For this review, take the finished solid that the model builds, in its own axes (mm). A direction names the side the tool comes from. Coordinates: 2 decimals unless noted, no trailing zeros. Order: outer loops, then holes, each group sorted by start corner. A loop starts at its lowest first (then second) coordinate and runs counter-clockwise, first axis right, second up. Notation, with made-up numbers: (-32, 14.5) -> (-1, 14.5) arc R30 ccw to (-1, 36.5) -> close; hole circle Ø4 at (-24, -24). An arc over 180 degrees is marked (long way). Return JSON: item names as keys, results as strings. Group by question number.
Item 1: Machinability: for faces 4 (the flat face through (-21.576, -30.4, 34.3)), 5 (the flat face through (0, -30.8, 0)), 6 (the flat face through (0, 1.336, 20)), 7 (the flat face through (0, -26, 33.65)), 8 (the flat face through (-21.576, -30.4, -34.3)), which of the approach directions +Z, -Z, +X, -X, +Y, -Y give a long, thin tool a straight path to every point of the face, cutting with its end or side? Answer none if there is none.
Item 2: Take a section at B-B (z = -38.75). Write out the cut boundary in (x, y) (3 decimals), then the cut area to 3 significant figures.
Item 3: Insertion check: pin 1 (8 mm diameter, centred on x = 4, z = 39.5, fed in from +Y); pin 2 (2 mm diameter, centred on x = -11, z = -9, fed in from +Y); pin 3 (0.7 mm diameter, centred on x = 2.5, z = -32, fed in from +Y). Each pin has a flat end and moves straight along its axis. Give the tip position at first contact, or say it passes through.
Item 4: For line 1 along X through (y, z) = (-31.1, 38.75) (3 decimals); line 2 along Y through (x, z) = (0, 16); line 3 along Y through (x, z) = (-16, -16), list the stretches that pass through material, from the lowest coordinate up.
Item 5: Draft analysis for pull direction Z (two halves, no side actions). For faces 1 (the cylindrical face through (13.947, -31.291, -40.505)), 2 (the flat face through (0, -30.15, 39)), 3 (the flat face through (0, -31, 43.7)), state which applies: +Z half, -Z half, draft (parallel to the pull), parting line (faces both ways), or undercut.
Item 6: Take a section at C-C (y = -27). Write out the cut boundary in (x, z).
Item 7: Take a section at A-A (z = 38.75). Write out the cut boundary in (x, y) (3 decimals), then the cut area to 3 significant figures.
Item 8: Take a section at D-D (x = 19). Write out the cut boundary in (y, z).
```python
from build123d import *

# Parameters (mm, degrees)
SKETCH1_W                = 46.2
SKETCH1_H                = 60
BOSS_EXTRUDE1_DEPTH      = 30.8
FILLET1_R                = 1.524
BOSS_EXTRUDE2_DEPTH      = 6
BOSS_EXTRUDE2_DEPTH_BACK = 12.07
SKETCH2_R                = 8.849999953
SKETCH3_R                = 5.849999953
CUT_EXTRUDE1_DEPTH       = 35.464
SKETCH4_R                = 8.8
BOSS_EXTRUDE3_DEPTH      = 11.6
SKETCH5_R                = 5.8
CUT_EXTRUDE2_DEPTH       = 59.86
SKETCH6_W                = 43.152
SKETCH6_H                = 5.5
BOSS_EXTRUDE4_DEPTH      = 1.4
BOSS_EXTRUDE5_DEPTH      = 43.152
SKETCH9_R                = 1.9
CUT_EXTRUDE3_DEPTH       = 14.1


with BuildPart() as part:
    # Sketch1 → Boss-Extrude1 (new, symmetric)
    with BuildSketch(Plane(origin=(0, 0, 0), x_dir=(1, 0, 0), z_dir=(0, 1, 0))):
        Rectangle(SKETCH1_W, SKETCH1_H)
    extrude(amount=BOSS_EXTRUDE1_DEPTH, both=True)

    # Fillet1
    fillet1_edges = [part.edges().sort_by_distance(p)[0] for p in [
        (-23.1, 30.8, 0),
        (0, 30.8, 30),
        (23.1, 30.8, 0),
        (0, -30.8, 30),
        (-23.1, -30.8, 0),
        (0, -30.8, -30),
        (23.1, -30.8, 0),
        (0, 30.8, -30),
        (23.1, 0, 30),
        (-23.1, 0, 30),
        (-23.1, 0, -30),
        (23.1, 0, -30),
    ]]
    fillet(fillet1_edges, radius=FILLET1_R)

    # Sketch2 → Boss-Extrude2 (add, two sides: drawn at the far end of the back side and taken through both)
    with BuildSketch(Plane(origin=(0, 30.8, 0), x_dir=(1, 0, 0), z_dir=(0, 1, 0)).offset(-BOSS_EXTRUDE2_DEPTH_BACK)):
        with Locations(Location((0, -20.545484859, 0), (0, 0, 270))):
            Circle(SKETCH2_R)
    extrude(amount=BOSS_EXTRUDE2_DEPTH + BOSS_EXTRUDE2_DEPTH_BACK)

    # Sketch3 → Cut-Extrude1 (cut)
    with BuildSketch(Plane(origin=(0, 36.8, 0), x_dir=(1, 0, 0), z_dir=(0, 1, 0))):
        with Locations(Location((0, -20.545484859, 0), (0, 0, 270))):
            Circle(SKETCH3_R)
    extrude(amount=-CUT_EXTRUDE1_DEPTH, mode=Mode.SUBTRACT)

    # Sketch4 → Boss-Extrude3 (add)
    with BuildSketch(Plane.XY.offset(30)):
        with Locations(Location((0, -6.2, 0), (0, 0, 180))):
            Circle(SKETCH4_R)
    extrude(amount=BOSS_EXTRUDE3_DEPTH)

    # Sketch5 → Cut-Extrude2 (cut)
    with BuildSketch(Plane.XY.offset(41.6)):
        with Locations((0, -6.2)):
            Circle(SKETCH5_R)
    extrude(amount=-CUT_EXTRUDE2_DEPTH, mode=Mode.SUBTRACT)

    # Sketch6 → Boss-Extrude4 (add)
    with BuildSketch(Plane.XY.offset(30)):
        with Locations((0, -26.526)):
            Rectangle(SKETCH6_W, SKETCH6_H)
    boss_extrude4 = extrude(amount=BOSS_EXTRUDE4_DEPTH)

    # Sketch8 → Boss-Extrude5 (add)
    with BuildSketch(Plane.ZY.offset(21.576)):
        Polygon((31.4, -32.4), (31.4, -22.595531019), (33.65, -22.595531019), (33.65, -30.15), (43.7, -30.15), (43.7, -32.4), align=None)
    boss_extrude5 = extrude(amount=-BOSS_EXTRUDE5_DEPTH)

    # Mirror1: Boss-Extrude4, Boss-Extrude5 across plane
    add(boss_extrude4.mirror(Plane.XY))
    add(boss_extrude5.mirror(Plane.XY))

    # Sketch9 → Cut-Extrude3 (cut)
    with BuildSketch(Plane.XZ.offset(32.4)):
        with Locations(Location((-14.675, 38.75, 0), (0, 0, 270))):
            Circle(SKETCH9_R)
        with Locations(Location((14.675, 38.75, 0), (0, 0, 270))):
            Circle(SKETCH9_R)
        with Locations(Location((14.675, -38.75, 0), (0, 0, 270))):
            Circle(SKETCH9_R)
        with Locations(Location((-14.675, -38.75, 0), (0, 0, 270))):
            Circle(SKETCH9_R)
    extrude(amount=-CUT_EXTRUDE3_DEPTH, mode=Mode.SUBTRACT)


solid = part.part
```
Findings below:
{
 "1": {"face 4": "+Z, -X, +Y, -Y", "face 5": "+X, -X, -Y", "face 6": "+Y", "face 7": "+Z, +X, -X", "face 8": "-Z, -X, +Y, -Y"},
 "2": {"outline": "(-21.576, -32.4) -> (-16.575, -32.4) -> (-16.575, -30.15) -> (-21.576, -30.15) -> close; (-12.775, -32.4) -> (12.775, -32.4) -> (12.775, -30.15) -> (-12.775, -30.15) -> close; (16.575, -32.4) -> (21.576, -32.4) -> (21.576, -30.15) -> (16.575, -30.15) -> close", "area": "80.0 mm2"},
 "3": {"pin 1": "stops at y = 2.6", "pin 2": "stops at y = 30.8", "pin 3": "stops at y = -22.6"},
 "4": {"line 1": "x = -21.576 to -16.575, -12.775 to 12.775, 16.575 to 21.576", "line 2": "y = -30.8 to -12, -0.4 to 1.34", "line 3": "y = -30.8 to 30.8"},
 "5": {"face 1": "undercut", "face 2": "draft", "face 3": "+Z half"},
 "6": {"outline": "(-23.1, -28.48) arc R1.52 ccw to (-21.58, -30) -> (-21.58, -33.65) -> (21.58, -33.65) -> (21.58, -30) arc R1.52 ccw to (23.1, -28.48) -> (23.1, 28.48) arc R1.52 ccw to (21.58, 30) -> (21.58, 33.65) -> (-21.58, 33.65) -> (-21.58, 30) arc R1.52 ccw to (-23.1, 28.48) -> close"},
 "7": {"outline": "(-21.576, -32.4) -> (-16.575, -32.4) -> (-16.575, -30.15) -> (-21.576, -30.15) -> close; (-12.775, -32.4) -> (12.775, -32.4) -> (12.775, -30.15) -> (-12.775, -30.15) -> close; circle Ø17.6 at (0, -6.2); (16.575, -32.4) -> (21.576, -32.4) -> (21.576, -30.15) -> (16.575, -30.15) -> close; hole circle Ø11.6 at (0, -6.2)", "area": "218 mm2"},
 "8": {"outline": "(-32.4, -43.7) -> (-30.15, -43.7) -> (-30.15, -33.65) -> (-22.6, -33.65) -> (-22.6, -31.4) -> (-23.78, -31.4) -> (-23.78, -30) -> (29.28, -30) arc R1.52 ccw to (30.8, -28.48) -> (30.8, 28.48) arc R1.52 ccw to (29.28, 30) -> (-23.78, 30) -> (-23.78, 31.4) -> (-22.6, 31.4) -> (-22.6, 33.65) -> (-30.15, 33.65) -> (-30.15, 43.7) -> (-32.4, 43.7) -> (-32.4, 31.4) -> (-29.28, 31.4) -> (-29.28, 30) arc R1.52 ccw to (-30.8, 28.48) -> (-30.8, -28.48) arc R1.52 ccw to (-29.28, -30) -> (-29.28, -31.4) -> (-32.4, -31.4) -> close"}
}
